The model under review builds one solid part; all positions refer to its coordinate system, in mm. A direction names the side the tool comes from. Round coordinates to 2 decimals unless told otherwise and drop trailing zeros. Loops run counter-clockwise (first coordinate to the right, second up) from the corner with the lowest first, then second, coordinate; pieces in that order, holes last. Notation, with made-up numbers: (67.25, 73.25) -> (107.25, 73.25) arc R14 cw to (107.25, 79.25) -> close; hole circle Ø10 at (46.25, 6.5). An arc over 180 degrees is marked (long way). Use a Markdown table: item, result. Add a question column.
1) Consider section B-B on x = 9. Give the boundary of the cut face in (y, z), plus the area to 3 significant figures.
2) Wall thickness on probe 1 along X at (y, z) = (-34, -0.5); probe 2 along Z at (x, y) = (5, -19); probe 3 along Z at (x, y) = (-26, -17): over which ranges is each line inside the solid? List them lowest first.
3) Consider section C-C on z = 5. Give the boundary of the cut face in (x, y).
4) Insertion check: pin 1 (2 mm diameter, centred on y = -22, z = -16.5, fed in from +X); pin 2 (12.5 mm diameter, centred on x = -12.5, z = -5, fed in from -Y); pin 3 (1.5 mm diameter, centred on x = 29, y = -25, fed in from +Z). Each pin has a flat end and moves straight along its axis. Give the tip position at first contact, or say it passes through.
5) Mouldability with a two-part tool opening along X and no side actions: class faces 3 (the cylindrical face through (32.505, -25.578, -19.963)), 4 (the cylindrical face through (34.28, -25.58, -21.78)), 5 (the cylindrical face through (-0.36, -3.62, -21.58)), 6 (the cylindrical face through (-32.663, -25.578, 19.805)) as released by +X, released by -X, zero draft, split by the parting line, or undercut.
6) For faces 1 (the cylindrical face through (-34.28, -3.62, 0.18)), 2 (the flat face through (0, -25, -22.86)), list the 3-axis set-ups (+Z, -Z, +X, -X, +Y, -Y) from which the entire face can be reached by the end or side of a thin tool; tool diameter is ignored.
7) Consider section D-D on y = -8. Give the boundary of the cut face in (x, z).
8) Consider section A-A on y = -30. Give the boundary of the cut face in (x, z), plus the area to 3 significant figures.
from build123d import *

# Parameters (mm, degrees)
F0_W     = 76.2
F0_H     = 50.8
F1_DEPTH = 38.1
F2_R     = 12.7
F3_R     = 12.7
F4_T     = -2.54


with BuildPart() as f1:
    # F0 (on Front) → F1 (new body)
    with BuildSketch(Plane.XZ):
        Rectangle(F0_W, F0_H)
    extrude(amount=F1_DEPTH)

    # F2
    f2_edges = [f1.edges().sort_by_distance(p)[0] for p in [
        (38.1, -19.05, 25.4),
        (38.1, -19.05, -25.4),
        (-38.1, -19.05, 25.4),
        (-38.1, -19.05, -25.4),
    ]]
    fillet(f2_edges, radius=F2_R)

    # F3
    f3_edges = [f1.edges().sort_by_distance(p)[0] for p in [
        (0, 0, 25.4),
    ]]
    fillet(f3_edges, radius=F3_R)

    # F4
    f4_openings = [f1.faces().sort_by_distance(p)[0] for p in [
        (0, -38.1, 0),
    ]]
    offset(amount=F4_T, openings=f4_openings)


solid = f1.part
Result set:
| question | item | result |
|---|---|---|
| 1 | outline | (-38.1, -25.4) -> (-12.7, -25.4) arc R12.7 ccw to (0, -12.7) -> (0, 12.7) arc R12.7 ccw to (-12.7, 25.4) -> (-38.1, 25.4) -> (-38.1, 22.86) -> (-12.7, 22.86) arc R10.16 cw to (-2.54, 12.7) -> (-2.54, -12.7) arc R10.16 cw to (-12.7, -22.86) -> (-38.1, -22.86) -> close |
| 1 | area | 285 mm2 |
| 2 | probe 1 | -38.1 to -35.56, 35.56 to 38.1 |
| 2 | probe 2 | -25.4 to -22.86, 22.86 to 25.4 |
| 2 | probe 3 | -25.39 to -22.84, 22.84 to 25.39 |
| 3 | outline | (-38.1, -38.1) -> (-35.56, -38.1) -> (-35.56, -12.7) arc R10.16 cw to (-25.4, -2.54) -> (25.4, -2.54) arc R10.16 cw to (35.56, -12.7) -> (35.56, -38.1) -> (38.1, -38.1) -> (38.1, -12.7) arc R12.7 ccw to (25.4, 0) -> (-25.4, 0) arc R12.7 ccw to (-38.1, -12.7) -> close |
| 4 | pin 1 | x = 37.79 |
| 4 | pin 2 | y = -2.54 |
| 4 | pin 3 | z = 25.08 |
| 5 | face 3 | undercut |
| 5 | face 4 | released by +X |
| 5 | face 5 | zero draft |
| 5 | face 6 | undercut |
| 6 | face 1 | +Z, -Z, -X, +Y |
| 6 | face 2 | -Y |
| 7 | outline | (-37.2, -12.7) arc R11.8 ccw to (-25.4, -24.5) -> (25.4, -24.5) arc R11.8 ccw to (37.2, -12.7) -> (37.2, 12.7) arc R11.8 ccw to (25.4, 24.5) -> (-25.4, 24.5) arc R11.8 ccw to (-37.2, 12.7) -> close; hole (-34.41, -12.7) arc R9.01 ccw to (-25.4, -21.71) -> (25.4, -21.71) arc R9.01 ccw to (34.41, -12.7) -> (34.41, 12.7) arc R9.01 ccw to (25.4, 21.71) -> (-25.4, 21.71) arc R9.01 ccw to (-34.41, 12.7) -> close |
| 8 | outline | (-38.1, -12.7) arc R12.7 ccw to (-25.4, -25.4) -> (25.4, -25.4) arc R12.7 ccw to (38.1, -12.7) -> (38.1, 12.7) arc R12.7 ccw to (25.4, 25.4) -> (-25.4, 25.4) arc R12.7 ccw to (-38.1, 12.7) -> close; hole (-35.56, -12.7) arc R10.16 ccw to (-25.4, -22.86) -> (25.4, -22.86) arc R10.16 ccw to (35.56, -12.7) -> (35.56, 12.7) arc R10.16 ccw to (25.4, 22.86) -> (-25.4, 22.86) arc R10.16 ccw to (-35.56, 12.7) -> close |
| 8 | area | 570 mm2 |
